Autodesk Inventor part; units mm, degrees
ref_plane "YZ Plane" through (0, 0, 0) normal (1, 0, 0) x (0, 1, 0)
ref_plane "XZ Plane" through (0, 0, 0) normal (0, 1, 0) x (-1, 0, 0)
ref_plane "XY Plane" through (0, 0, 0) normal (0, 0, 1) x (1, 0, 0)
sketch "Sketch1" plane through (0, 0, 0) normal (0, 0, 1) x (1, 0, 0)
  circle A0 centre (0, 0) radius 45.212
  dimension "d0" = 90.424
extrude "Extrusion1" add sketch "Sketch1" along normal blind 4.7625
sketch "Sketch2" plane through (0, 0, 4.7625) normal (0, 0, 1) x (1, 0, 0)
  line L0 (0, 0) -> (0, 41.91)
  circle A0 centre (0, 41.91) radius 1.8415
  circle A1 centre (-36.2951, 20.955) radius 1.8415
  circle A2 centre (-36.2951, -20.955) radius 1.8415
  circle A3 centre (0, -41.91) radius 1.8415
  circle A4 centre (36.2951, -20.955) radius 1.8415
  circle A5 centre (36.2951, 20.955) radius 1.8415
  dimension "d3" = 41.91
  dimension "d4" = 3.683
  dimension "d7" = 360
extrude "Extrusion2" cut sketch "Sketch2" against normal blind 4.7625
sketch "Sketch4" plane through (0, 0, 4.7625) normal (0, 0, 1) x (1, 0, 0)
  circle A0 centre (36.2951, -20.955) radius 1.8415
  circle A1 centre (-36.2951, -20.955) radius 1.8415
  circle A2 centre (0, 41.91) radius 1.8415
  circle A3 centre (-36.2951, 20.955) radius 1.8415
  circle A4 centre (0, -41.91) radius 1.8415
  circle A5 centre (36.2951, 20.955) radius 1.8415
  circle A6 centre (0, 0) radius 45.212
  circle A7 centre (0, 0) radius 36.83
  dimension "d17" = 73.66
extrude "Extrusion4" cut sketch "Sketch4" against normal blind 25.4 contours A7
properties part number "foreElectronicsSealingDisc" material "Aluminum 6061"
Work out the finished part from the listing and answer in its coordinate system (mm). Give positions to 0.01 mm unless a question says otherwise; leave off trailing zeros. Loops run counter-clockwise (first coordinate to the right, second up) from the corner with the lowest first, then second, coordinate; pieces in that order, holes last. Notation, with made-up numbers: (40.5, -26) -> (45.5, -26) arc R11 cw to (45.5, -15) -> close; hole circle Ø6 at (-12.75, 43.5). An arc over 180 degrees is marked (long way). Use a Markdown table: item, result. Add a question column.
1) The part is cut by section B-B, the plane x = 0. Determine the outline of the cut face in (y, z).
2) For a pull along X with two mould halves and no side action, classify faces 1 (the cylindrical face through (43.124, -13.58, 2.348)), 2 (the flat face through (6, -37, 0)), 3 (the cylindrical face through (-34.54, 21.51, 2.41)), 4 (the cylindrical face through (-29.227, -22.41, 2.415)) as +X half, -X half, draft (parallel to the pull), parting line (faces both ways), or undercut.
3) Each of these flat-tipped pins is pushed along its axis until it touches: P1, Ø2, axis at x = -18, z = 0.5, coming from the +Y side; P2, Ø3.5, axis at x = 36.3, y = -20.96, coming from the +Z side. Where does it stop, or does it pass through?
4) The part is cut by section A-A, the plane y = 0. Determine the outline of the cut face in (x, z).
5) Consider line 1 along Y through (x, z) = (0, 1.65); line 2 along Y through (x, z) = (37, 0.55); line 3 along X through (y, z) = (22.5, 3.15). Determine where each line is inside the solid, lowest interval first.
6) The part is cut by section D-D, the plane z = 2.25. Determine the outline of the cut face in (x, y) (1 decimal).
7) The part is cut by section C-C, the plane x = -25.5. Determine the outline of the cut face in (y, z).
Reported:
| question | item | result |
|---|---|---|
| 1 | outline | (-45.21, 0) -> (-43.75, 0) -> (-43.75, 4.76) -> (-45.21, 4.76) -> close; (-40.07, 0) -> (-36.83, 0) -> (-36.83, 4.76) -> (-40.07, 4.76) -> close; (36.83, 0) -> (40.07, 0) -> (40.07, 4.76) -> (36.83, 4.76) -> close; (43.75, 0) -> (45.21, 0) -> (45.21, 4.76) -> (43.75, 4.76) -> close |
| 2 | face 1 | parting line |
| 2 | face 2 | draft |
| 2 | face 3 | undercut |
| 2 | face 4 | undercut |
| 3 | P1 | stops at y = 41.89 |
| 3 | P2 | passes through |
| 4 | outline | (-45.21, 0) -> (-36.83, 0) -> (-36.83, 4.76) -> (-45.21, 4.76) -> close; (36.83, 0) -> (45.21, 0) -> (45.21, 4.76) -> (36.83, 4.76) -> close |
| 5 | line 1 | y = -45.21 to -43.75, -40.07 to -36.83, 36.83 to 40.07, 43.75 to 45.21 |
| 5 | line 2 | y = -25.98 to -22.66, -19.25 to 19.25, 22.66 to 25.98 |
| 5 | line 3 | x = -39.22 to -37.3, -35.29 to -29.16, 29.16 to 35.29, 37.3 to 39.22 |
| 6 | outline | circle Ø90.4 at (0, 0); hole circle Ø3.7 at (-36.3, -21); hole circle Ø3.7 at (-36.3, 21); hole circle Ø73.7 at (0, 0); hole circle Ø3.7 at (0, -41.9); hole circle Ø3.7 at (0, 41.9); hole circle Ø3.7 at (36.3, -21); hole circle Ø3.7 at (36.3, 21) |
| 7 | outline | (-37.33, 0) -> (-26.57, 0) -> (-26.57, 4.76) -> (-37.33, 4.76) -> close; (26.57, 0) -> (37.33, 0) -> (37.33, 4.76) -> (26.57, 4.76) -> close |
